CAD build for the part. Positions are in the model's coordinates, mm. A direction names the side the tool comes from. Coordinates: 2 decimals unless noted, no trailing zeros. Write each loop counter-clockwise with the first axis right and the second up, starting at its lowest first coordinate (ties: lowest second). Pieces come first, ordered by that corner, then holes. Notation, with made-up numbers: (-17.75, 48.25) -> (9.25, 48.25) arc R11 cw to (9.25, 56.25) -> close; hole circle Ø4 at (89, 8.25). An arc over 180 degrees is marked (long way). Answer as CSV lines item,"result".
Autodesk Fusion 360 part; units mm, degrees
sketch "Sketch3" plane through (0, 0, 0) normal (0, 1, 0) x (1, 0, 0)
  circle A0 centre (12.4, 0) radius 8
  line L0 (-22.7, 10.2) -> (-22.7, -10.2)
  line L1 (-22.7, -10.2) -> (22.7, -10.2)
  line L2 (22.7, -10.2) -> (22.7, 10.2)
  line L3 (22.7, 10.2) -> (-22.7, -10.2) construction
  line L4 (-22.7, 10.2) -> (22.7, -10.2) construction
  circle A1 centre (-12.5, 0) radius 8
  line L5 (4.5, -4.75) -> (-4.5, -4.75)
  line L6 (-5.5, -5.75) -> (-5.5, -8.25)
  line L7 (-4.5, -9.25) -> (4.5, -9.25)
  line L8 (5.5, -8.25) -> (5.5, -5.75)
  line L9 (5.5, -4.75) -> (-5.5, -9.25) construction
  line L10 (-5.5, -4.75) -> (5.5, -9.25) construction
  arc A2 (-5.5, -8.25) -> (-4.5, -9.25) centre (-4.5, -8.25) ccw
  arc A3 (4.5, -9.25) -> (5.5, -8.25) centre (4.5, -8.25) ccw
  arc A4 (5.5, -5.75) -> (4.5, -4.75) centre (4.5, -5.75) ccw
  arc A5 (-4.5, -4.75) -> (-5.5, -5.75) centre (-4.5, -5.75) ccw
  line L11 (15.0179, 10.2) -> (15.0179, 54)
  line L12 (15.0179, 54) -> (-14.9821, 54)
  line L13 (-14.9821, 54) -> (-14.9821, 10.2)
  line L14 (22.7, 10.2) -> (15.0179, 10.2)
  line L15 (-14.9821, 10.2) -> (-22.7, 10.2)
  point P0 (0, -7)
  dimension "d8" = 16
  dimension "d10" = 45.4
  dimension "d11" = 20.4
  dimension "d12" = 16
  dimension "d13" = 11
  dimension "d14" = 4.5
  dimension "d15" = 1
  dimension "d16" = 1
  dimension "d17" = 30
  dimension "d18" = 43.8
sketch "Sketch4" plane through (0, 0, 0) normal (0, 1, 0) x (1, 0, 0)
  line L0 (-15, 54) -> (15, 54)
  line L1 (15, 54) -> (15, 51)
  line L2 (15, 51) -> (-15, 51)
  line L3 (-15, 51) -> (-15, 54)
extrude "Extrude1" add sketch "Sketch3" along normal blind 3
extrude "Extrude2" add sketch "Sketch4" against normal blind 20
sketch "Sketch1" plane through (0, 0, 0) normal (0, 1, 0) x (1, 0, 0)
sketch "Sketch2" plane through (0, 0, 0) normal (0, 1, 0) x (1, 0, 0)
Item 1: Saw through at B-B on z = 0. Give the cut face in (x, y), and give its area (3 significant figures).
Answer below:
outline,"(-22.7, 0) -> (-20.5, 0) -> (-20.5, 3) -> (-22.7, 3) -> close; (-4.5, 0) -> (4.4, 0) -> (4.4, 3) -> (-4.5, 3) -> close; (20.4, 0) -> (22.7, 0) -> (22.7, 3) -> (20.4, 3) -> close"
area,"40.2 mm2"
Item 2: Flat gauge pins, fed straight in: pin 1 (10 mm diameter, centred on x = -2.5, y = -7.5, fed in from +Z); pin 2 (2.5 mm diameter, centred on y = -7, z = -52, fed in from +X); pin 3 (2.5 mm diameter, centred on x = -20.5, y = 1.5, fed in from -Z). Where does each tip first touch, or does it go through?
Answer below:
pin 1,"stops at z = -51"
pin 2,"stops at x = 15"
pin 3,"stops at z = -10.2"
Item 3: Saw through at A-A on x = -12.5. Give the cut face in (y, z).
Answer below:
outline,"(-20, -54) -> (3, -54) -> (3, -8) -> (0, -8) -> (0, -51) -> (-20, -51) -> close; (0, 8) -> (3, 8) -> (3, 10.2) -> (0, 10.2) -> close"
Item 4: Saw through at C-C on y = 0.75. Give the cut face in (x, z), and give its area (3 significant figures).
Answer below:
outline,"(-22.7, -10.2) -> (-14.98, -10.2) -> (-14.98, -54) -> (15.02, -54) -> (15.02, -10.2) -> (22.7, -10.2) -> (22.7, 10.2) -> (-22.7, 10.2) -> close; hole circle Ø16 at (-12.5, 0); hole (-5.5, 5.75) arc R1 ccw to (-4.5, 4.75) -> (4.5, 4.75) arc R1 ccw to (5.5, 5.75) -> (5.5, 8.25) arc R1 ccw to (4.5, 9.25) -> (-4.5, 9.25) arc R1 ccw to (-5.5, 8.25) -> close; hole circle Ø16 at (12.4, 0)"
area,"1,790 mm2"
Item 5: Two-plate mould, pull along X, no slides. Class faces 1 (the flat face through (22.7, 1, 0)), 2 (the cylindrical face through (4.408, 1.479, 0.352)), 3 (the flat face through (-22.7, 1, 0)), 4 (the cylindrical face through (-14.23, 1.48, -7.81)): pulls with the +X half, pulls with the -X half, needs draft (parallel to the pull), parting line crosses it, or undercut.
Answer below:
face 1,"pulls with the +X half"
face 2,"undercut"
face 3,"pulls with the -X half"
face 4,"undercut"
Item 6: Wall check: line 1 (X direction, y = 1.4, z = 0); line 2 (Z direction, x = -8.5, y = -12.25); line 3 (Z direction, x = -12.5, y = 1.35). Give the ranges that are in metal, low to high. Write a range as from..to.
Answer below:
line 1,"x = -22.7..-20.5, -4.5..4.4, 20.4..22.7"
line 2,"z = -54..-51"
line 3,"z = -54..-8, 8..10.2"
Item 7: 3-axis set-ups, long thin cutter, end or side, ignore diameter. For faces 5 (the flat face through (15.018, 1, -32)), 6 (the flat face through (-19, 1, -10.2)), 7 (the flat face through (-5.5, 1, 7)), 8 (the flat face through (0, -10, -51)): which of +Z, -Z, +X, -X, +Y, -Y reach the whole face in a straight line?
Answer below:
face 5,"-Z, +X, +Y, -Y"
face 6,"-Z, -X, +Y, -Y"
face 7,"+Y, -Y"
face 8,"+Z, +X, -X, -Y"
Item 8: Saw through at D-D on x = 2.5. Give the cut face in (y, z).
Answer below:
outline,"(-20, -54) -> (3, -54) -> (3, 4.75) -> (0, 4.75) -> (0, -51) -> (-20, -51) -> close; (0, 9.25) -> (3, 9.25) -> (3, 10.2) -> (0, 10.2) -> close"
